Read the model definition and answer for the solid it produces. Units are mm, in the model's axes. Coordinates: 2 decimals unless noted, no trailing zeros. Loops run counter-clockwise (first coordinate to the right, second up) from the corner with the lowest first, then second, coordinate; pieces in that order, holes last. Notation, with made-up numbers: (62, 18) - (121, 18) arc R25 cw to (121, 55) - close; hole circle Ø3 at (89.25, -30.5). An arc over 180 degrees is marked (long way). One line per item, written item: value. Start each with the question number.
from build123d import *

# Parameters (mm, degrees)
SKETCH1_R           = 1.5
SKETCH1_R_2         = 7
BOSS_EXTRUDE1_DEPTH = 1


with BuildPart() as part:
    # Sketch1 → Boss-Extrude1 (new body)
    with BuildSketch(Plane(origin=(0, 0, 0), x_dir=(1, 0, 0), z_dir=(0, 1, 0))):
        with BuildLine():
            Line((-2.365441422, 14.812315379), (-29.157696095, 10.533746677))
            ThreePointArc((-29.157696095, 10.533746677), (-29.760820641, 10.195221197), (-30, 9.546258985))
            Line((-30, 9.546258985), (-30, 1.658312395))
            ThreePointArc((-30, 1.658312395), (-30.5, 0), (-30, -1.658312395))
            Line((-30, -1.658312395), (-30, -9.546258985))
            ThreePointArc((-30, -9.546258985), (-29.760820641, -10.195221197), (-29.157696095, -10.533746677))
            Line((-29.157696095, -10.533746677), (-2.365441422, -14.812315379))
            ThreePointArc((-2.365441422, -14.812315379), (0, -15), (2.365441422, -14.812315379))
            Line((2.365441422, -14.812315379), (29.157696095, -10.533746677))
            ThreePointArc((29.157696095, -10.533746677), (29.760820641, -10.195221197), (30, -9.546258985))
            Line((30, -9.546258985), (30, -1.658312395))
            ThreePointArc((30, -1.658312395), (30.5, 0), (30, 1.658312395))
            Line((30, 1.658312395), (30, 9.546258985))
            ThreePointArc((30, 9.546258985), (29.760820641, 10.195221197), (29.157696095, 10.533746677))
            Line((29.157696095, 10.533746677), (2.365441422, 14.812315379))
            ThreePointArc((2.365441422, 14.812315379), (0, 15), (-2.365441422, 14.812315379))
        make_face()
        with Locations(Location((8.838834765, 8.838834765, 0), (0, 0, 270))):
            Circle(SKETCH1_R, mode=Mode.SUBTRACT)
        with Locations(Location((-8.838834765, -8.838834765, 0), (0, 0, 270))):
            Circle(SKETCH1_R, mode=Mode.SUBTRACT)
        with Locations(Location((8.838834765, -8.838834765, 0), (0, 0, 270))):
            Circle(SKETCH1_R, mode=Mode.SUBTRACT)
        with Locations(Location((0, 0, 0), (0, 0, 270))):
            Circle(SKETCH1_R_2, mode=Mode.SUBTRACT)
        with Locations(Location((-8.838834765, 8.838834765, 0), (0, 0, 270))):
            Circle(SKETCH1_R, mode=Mode.SUBTRACT)
        with Locations(Location((-27.5, 0, 0), (0, 0, 270))):
            Circle(SKETCH1_R, mode=Mode.SUBTRACT)
        with Locations(Location((27.5, 0, 0), (0, 0, 270))):
            Circle(SKETCH1_R, mode=Mode.SUBTRACT)
    extrude(amount=BOSS_EXTRUDE1_DEPTH)


solid = part.part
1) Section C-C, the plane y = 0.75 is taken. Determine the outline of the cut face in (x, z).
2) Flat-ended cylindrical pins translate along their axes: P1, Ø0.5, axis at y = 0.5, z = 5, coming from the -X side; P2, Ø5, axis at x = 0, z = 5.5, coming from the -Y side. Find the tip coordinate at first contact, or state that the pin passes through.
3) Section D-D, the plane z = -4 is taken. Determine the outline of the cut face in (x, y).
4) Straight lines are drawn through the part: L1, parallel to X at y = 0.65, z = 6.25; L2, parallel to X at y = 0.65, z = 7.75; L3, parallel to Z at x = -11, y = 0.25. For each, find the intervals that lie inside material, in ascending order.
5) Section A-A, the plane z = 0 is taken. Determine the outline of the cut face in (x, y), and give its area (3 significant figures).
6) Section B-B, the plane x = 0 is taken. Determine the outline of the cut face in (y, z), and give its area (3 significant figures).
7) Determine the mould class of faces 1 (the flat face through (15.6, 0.5, 12.7)), 2 (the cylindrical face through (-10.3, 0.5, 8.5)), 3 (the cylindrical face through (-9.75, 0.49, -10.03)), 4 (the flat face through (-7.2, 1, -0.2)) for opening direction X: released by +X, released by -X, zero draft, split by the parting line, or undercut.
Answer below:
1. outline: (-30, -9.55) arc R1 ccw to (-29.16, -10.53) - (-2.37, -14.81) arc R15 ccw to (2.37, -14.81) - (29.16, -10.53) arc R1 ccw to (30, -9.55) - (30, -1.66) arc R3 ccw to (30, 1.66) - (30, 9.55) arc R1 ccw to (29.16, 10.53) - (2.37, 14.81) arc R15 ccw to (-2.37, 14.81) - (-29.16, 10.53) arc R1 ccw to (-30, 9.55) - (-30, 1.66) arc R3 ccw to (-30, -1.66) - close; hole circle Ø3 at (-27.5, 0); hole circle Ø3 at (-8.84, -8.84); hole circle Ø3 at (-8.84, 8.84); hole circle Ø14 at (0, 0); hole circle Ø3 at (8.84, -8.84); hole circle Ø3 at (8.84, 8.84); hole circle Ø3 at (27.5, 0)
2. P1: x = -30
2. P2: y = 0
3. outline: (-30, 0) - (-5.74, 0) - (-5.74, 1) - (-30, 1) - close; (5.74, 0) - (30, 0) - (30, 1) - (5.74, 1) - close
4. L1: -30 to -3.15, 3.15 to 30
4. L2: -30 to -9.87, -7.81 to 7.81, 9.87 to 30
4. L3: -13.43 to 13.43
5. outline: (-30.5, 0) - (-29, 0) - (-29, 1) - (-30.5, 1) - close; (-26, 0) - (-7, 0) - (-7, 1) - (-26, 1) - close; (7, 0) - (26, 0) - (26, 1) - (7, 1) - close; (29, 0) - (30.5, 0) - (30.5, 1) - (29, 1) - close
5. area: 41.0 mm2
6. outline: (0, -15) - (1, -15) - (1, -7) - (0, -7) - close; (0, 7) - (1, 7) - (1, 15) - (0, 15) - close
6. area: 16.0 mm2
7. face 1: released by +X
7. face 2: undercut
7. face 3: undercut
7. face 4: zero draft
